```python
from build123d import *

# Parameters (mm, degrees)
SKETCH1_W           = 38.1
SKETCH1_H           = 25.4
BOSS_EXTRUDE1_DEPTH = 8
SKETCH2_W           = 5
SKETCH2_H           = 8
BOSS_EXTRUDE2_DEPTH = 10
SKETCH3_R           = 2
CUT_EXTRUDE1_DEPTH  = 30
LPATTERN1_COUNT     = 2
LPATTERN1_PITCH     = 33.1


with BuildPart() as part:
    # Sketch1 → Boss-Extrude1 (new body)
    with BuildSketch(Plane(origin=(0, 0, 0), x_dir=(1, 0, 0), z_dir=(0, 1, 0))):
        with Locations((19.05, 12.7)):
            Rectangle(SKETCH1_W, SKETCH1_H)
    extrude(amount=BOSS_EXTRUDE1_DEPTH)

    # Sketch2 → Boss-Extrude2 (add)
    with BuildSketch(Plane.XY):
        with Locations((35.6, 4)):
            Rectangle(SKETCH2_W, SKETCH2_H)
    boss_extrude2 = extrude(amount=BOSS_EXTRUDE2_DEPTH)

    # Sketch3 → Cut-Extrude1 (cut)
    with BuildSketch(Plane.ZY.offset(-33.1)):
        with Locations((5, 4)):
            Circle(SKETCH3_R)
    cut_extrude1 = extrude(amount=-CUT_EXTRUDE1_DEPTH, mode=Mode.SUBTRACT)

    # LPattern1: Boss-Extrude2, Cut-Extrude1 ×2
    with Locations(*[(-i * LPATTERN1_PITCH, 0, 0) for i in range(1, LPATTERN1_COUNT)]):
        add(boss_extrude2)
        add(cut_extrude1, mode=Mode.SUBTRACT)


solid = part.part
```
Could you check a few things on this model? Use its own coordinates, in mm. A direction names the side the tool comes from. Coordinates: 2 decimals unless noted, no trailing zeros. Write each loop counter-clockwise with the first axis right and the second up, starting at its lowest first coordinate (ties: lowest second). Pieces come first, ordered by that corner, then holes. Notation, with made-up numbers: (-39, -21) -> (4, -21) arc R24 cw to (4, 10) -> close; hole circle Ø8 at (53.25, -4.5). An arc over 180 degrees is marked (long way). Write item = value, one per line. Start each with the question number.
(1) We'd pull the mould along X, two halves only. Please class faces 3 (the face through (36, 4, 10)), 4 (the face through (0, 4, -8)), 5 (the face through (33.1, 6, 4)), 6 (the face through (38.1, 4, -8)): released by +X, released by -X, zero draft, split by the parting line, or undercut.
(2) Will these pins go through, and if not, where does the flat tip stop? pin 1 (4 mm diameter, centred on x = 22.5, y = 5.5, fed in from +Z); pin 2 (4.5 mm diameter, centred on y = 4, z = 5, fed in from +X).
(3) I want a section at D-D (z = 5). Please give me the cut outline in (x, y).
(4) I want a section at A-A (z = 1). Please give me the cut outline in (x, y), plus the area to 3 significant figures.
(5) Which directions (+Z, -Z, +X, -X, +Y, -Y) give clear straight access to the entire face, cutting with the end or side of a thin tool? Please do faces 1 (the face through (5, 6, 4)), 2 (the face through (35.6, 2.8, 3.4)).
(6) I need wall thicknesses on line 1 (X direction, y = 1.5, z = 4.5); line 2 (Y direction, x = 1, z = 5); line 3 (Z direction, x = 14.5, y = 3.25). Which ranges of each line are inside material? Lowest first, please. Write a range as [from, to].
(7) I want a section at C-C (x = 34.5). Please give me the cut outline in (y, z).
(8) I want a section at B-B (y = 4). Please give me the cut outline in (x, z), plus the area to 3 significant figures.
Result set:
q1.face_3 = zero draft
q1.face_4 = released by -X
q1.face_5 = undercut
q1.face_6 = released by +X
q2.pin_1 = 0
q2.pin_2 = 38.1
q3.outline = (0, 0) -> (5, 0) -> (5, 2) -> (0, 2) -> close; (0, 6) -> (5, 6) -> (5, 8) -> (0, 8) -> close; (33.1, 0) -> (38.1, 0) -> (38.1, 2) -> (33.1, 2) -> close; (33.1, 6) -> (38.1, 6) -> (38.1, 8) -> (33.1, 8) -> close
q4.outline = (0, 0) -> (5, 0) -> (5, 8) -> (0, 8) -> close; (33.1, 0) -> (38.1, 0) -> (38.1, 8) -> (33.1, 8) -> close
q4.area = 80.0 mm2
q5.face_1 = +Z, +Y, -Y
q5.face_2 = +X, -X
q6.line_1 = [0, 5], [33.1, 38.1]
q6.line_2 = [0, 2], [6, 8]
q6.line_3 = [-25.4, 0]
q7.outline = (0, -25.4) -> (8, -25.4) -> (8, 10) -> (0, 10) -> close; hole circle Ø4 at (4, 5)
q8.outline = (0, -25.4) -> (38.1, -25.4) -> (38.1, 3) -> (33.1, 3) -> (33.1, 0) -> (5, 0) -> (5, 3) -> (0, 3) -> close; (0, 7) -> (5, 7) -> (5, 10) -> (0, 10) -> close; (33.1, 7) -> (38.1, 7) -> (38.1, 10) -> (33.1, 10) -> close
q8.area = 1,030 mm2
